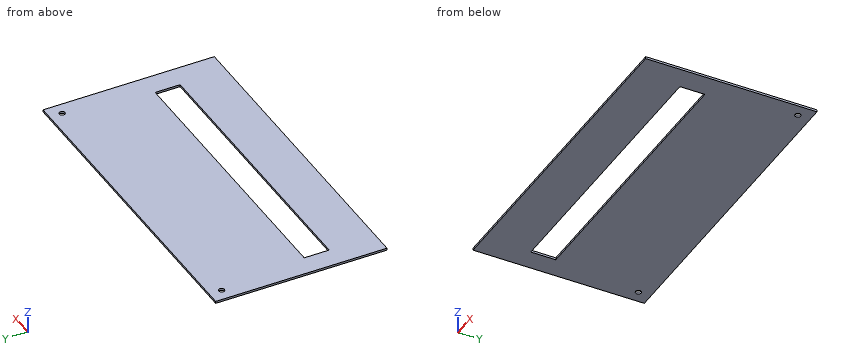
from build123d import *

# Parameters (mm, degrees)
SKETCH1_W           = 457.2
SKETCH1_H           = 240
BOSS_EXTRUDE1_DEPTH = 3
SKETCH2_R           = 4
CUT_EXTRUDE1_DEPTH  = 259.199457784
SKETCH3_W           = 394.7
SKETCH3_H           = 35
CUT_EXTRUDE2_DEPTH  = 259.199457784


with BuildPart() as part:
    # Sketch1 → Boss-Extrude1 (new body)
    with BuildSketch(Plane.XY):
        Rectangle(SKETCH1_W, SKETCH1_H)
    extrude(amount=BOSS_EXTRUDE1_DEPTH)

    # Sketch2 → Cut-Extrude1 (cut, through all)
    with BuildSketch(Plane.XY.offset(3)):
        with Locations((-211.1, 102.5)):
            Circle(SKETCH2_R)
        with Locations((211.1, 102.5)):
            Circle(SKETCH2_R)
    extrude(amount=-CUT_EXTRUDE1_DEPTH, mode=Mode.SUBTRACT)

    # Sketch3 → Cut-Extrude2 (cut, through all)
    with BuildSketch(Plane.XY.offset(3)):
        with Locations((-1.25, -37.4)):
            Rectangle(SKETCH3_W, SKETCH3_H)
    extrude(amount=-CUT_EXTRUDE2_DEPTH, mode=Mode.SUBTRACT)


solid = part.part
Geometry check sheet. Reference: the model listing, model coordinates, mm. Give positions to 0.01 mm unless a question says otherwise; leave off trailing zeros. Write each loop counter-clockwise with the first axis right and the second up, starting at its lowest first coordinate (ties: lowest second). Pieces come first, ordered by that corner, then holes. Notation, with made-up numbers: M 29,-2.5 L 44,-2.5 A22 cw 44,27.5 Z; hole C 6.5,30.25 d1. An arc over 180 degrees is marked long. Answer as CSV lines item,"result". Start each with the question number.
Q1. Material ranges on L1, parallel to X at y = 102, z = 0.1; L2, parallel to Y at x = -61, z = 1.4; L3, parallel to Y at x = 211.1, z = 1.55, recorded low to high.
Q2. Section check B-B, the plane x = 150.5. Record the cut outline in (y, z).
Q3. Section check C-C, the plane z = 0.9. Record the cut outline in (x, y).
Q4. Section check A-A, the plane y = -39.5. Record the cut outline in (x, z), then the cut area to 4 significant figures.
Geometry says:
1,L1,"-228.6 to -215.07, -207.13 to 207.13, 215.07 to 228.6"
1,L2,"-120 to -54.9, -19.9 to 120"
1,L3,"-120 to 98.5, 106.5 to 120"
2,outline,"M -120,0 L -54.9,0 L -54.9,3 L -120,3 Z; M -19.9,0 L 120,0 L 120,3 L -19.9,3 Z"
3,outline,"M -228.6,-120 L 228.6,-120 L 228.6,120 L -228.6,120 Z; hole C -211.1,102.5 d8; hole M -198.6,-54.9 L 196.1,-54.9 L 196.1,-19.9 L -198.6,-19.9 Z; hole C 211.1,102.5 d8"
4,outline,"M -228.6,0 L -198.6,0 L -198.6,3 L -228.6,3 Z; M 196.1,0 L 228.6,0 L 228.6,3 L 196.1,3 Z"
4,area,"187.5 mm^2"
